The listing builds one solid part. Answer for the finished solid, in the listing's coordinates (mm). Coordinates: 2 decimals unless noted, no trailing zeros. Order: outer loops, then holes, each group sorted by start corner. A loop starts at its lowest first (then second) coordinate and runs counter-clockwise, first axis right, second up. Notation, with made-up numbers: (56, -9) - (73, -9) arc R16 cw to (73, -1) - close; hole circle Ø5 at (3, 66). An arc over 180 degrees is marked (long way). Use one line per item in the form item = value. Start each with the question number.
Item 1: The mould has two halves that part along Y. Classify faces 1 (the cylindrical face through (-20.58, 15.62, -3.47)), 2 (the conical face through (8.67, -12.63, 8.05)), 3 (the flat face through (-24, -13.43, -8.98)): released by +Y, released by -Y, zero draft, split by the parting line, or undercut.
Item 2: Each of these flat-tipped pins is pushed along its axis until it touches: pin 1 Ø8 at (y, z) = (-2.5, -5) entering from +X; pin 2 Ø2 at (x, z) = (1.5, -9) entering from +Y; pin 3 Ø5 at (x, y) = (1, -8.5) entering from +Z. Where does it stop, or does it pass through?
Item 3: Section A-A, the plane x = -12.5 is taken. Write down the section's boundary in (y, z).
Item 4: Consider line 1 along Y through (x, z) = (-21.75, 0); line 2 along Y through (x, z) = (12.5, 9); line 3 along Z through (x, y) = (23, 0.5). Determine where each line is inside the solid, lowest interval first. Write a range as [from, to].
Item 5: Section B-B, the plane x = -4 is taken. Write down the section's boundary in (y, z).
from build123d import *


with BuildPart() as part:
    # Sketch1 → Revolve1 (revolve)
    with BuildSketch(Plane.XY, mode=Mode.PRIVATE) as revolve1_sk:
        with BuildLine():
            Line((-2, 13), (34.158093272, 5.887174193))
            ThreePointArc((34.158093272, 5.887174193), (37.634034939, 3.811262282), (39, 0))
            Line((39, 0), (43, 0))
            ThreePointArc((43, 0), (40.723391565, 6.352103804), (34.930155453, 9.811956988))
            Line((34.930155453, 9.811956988), (-16.860823192, 20))
            Line((-16.860823192, 20), (-24, 20))
            Line((-24, 20), (-24, 16))
            Line((-24, 16), (-17.250518254, 16))
            Line((-17.250518254, 16), (-2, 13))
        make_face()
    revolve(revolve1_sk.sketch.rotate(Axis((39, 0, 0), (1, 0, 0)), 90), axis=Axis((39, 0, 0), (1, 0, 0)))


solid = part.part
Response:
q1.face_1 = undercut
q1.face_2 = split by the parting line
q1.face_3 = zero draft
q2.pin_1 = 42.87
q2.pin_2 = 14.35
q2.pin_3 = 15.49
q3.outline = circle Ø38.28 at (0, 0); hole circle Ø30.13 at (0, 0)
q4.line_1 = [-20, -16], [16, 20]
q4.line_2 = [-11.02, -4.69], [4.69, 11.02]
q4.line_3 = [-12.15, -8.07], [8.07, 12.15]
q5.outline = circle Ø34.94 at (0, 0); hole circle Ø26.79 at (0, 0)
